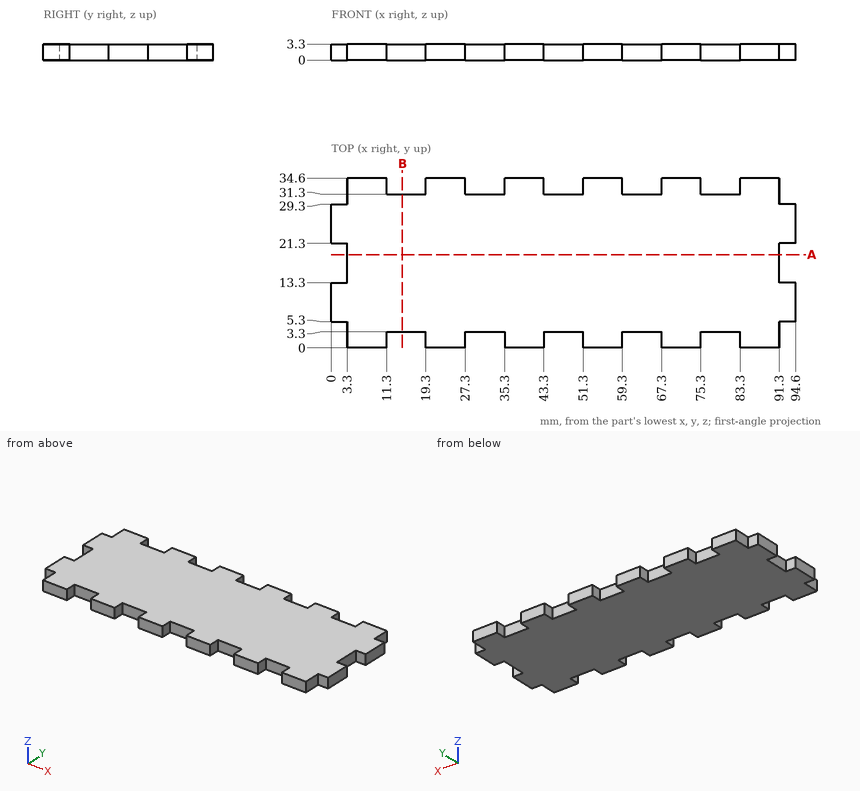
Study the drawing (mm; zero at the part's minimum x, y, z) and answer. Give positions to 0.01 mm unless a question says otherwise; leave off trailing zeros. Write each loop counter-clockwise with the first axis right and the second up, starting at its lowest first coordinate (ties: lowest second). Pieces come first, ordered by that corner, then holes. Notation, with made-up numbers: M 84.5,-26 L 135.5,-26 A11 ccw 135.5,-18 Z; hole C 45,-10 d6. An arc over 180 degrees is marked long. Put each result on its own line as item: value. Start each with the question number.
1. Each of these flat-tipped pins is pushed along its axis until it touches: pin 1 Ø1.6 at (x, z) = (63, 1) entering from -Y; pin 2 Ø1 at (x, z) = (93, 1.5) entering from -Y; pin 3 Ø1.5 at (y, z) = (19.5, 0.5) entering from +X. Where does it stop, or does it pass through?
2. Consider line 1 along X through (y, z) = (33, 0.8); line 2 along X through (y, z) = (30.5, 0.8); line 3 along Y through (x, z) = (46.5, 2.9). Determine where each line is inside the solid, lowest interval first.
3. The part is cut by section A-A, the plane y = 19. Give the vertices of the cut face in (x, z), and give its area (3 significant figures).
4. The part is cut by section B-B, the plane x = 14.5. Give the vertices of the cut face in (y, z).
Final values:
1. pin 1: stops at y = 3.3
1. pin 2: stops at y = 5.3
1. pin 3: stops at x = 91.3
2. line 1: x = 3.3 to 11.3, 19.3 to 27.3, 35.3 to 43.3, 51.3 to 59.3, 67.3 to 75.3, 83.3 to 91.3
2. line 2: x = 3.3 to 91.3
2. line 3: y = 3.3 to 31.3
3. outline: M 3.3,0 L 91.3,0 L 91.3,3.3 L 3.3,3.3 Z
3. area: 290 mm²
4. outline: M 3.3,0 L 31.3,0 L 31.3,3.3 L 3.3,3.3 Z
